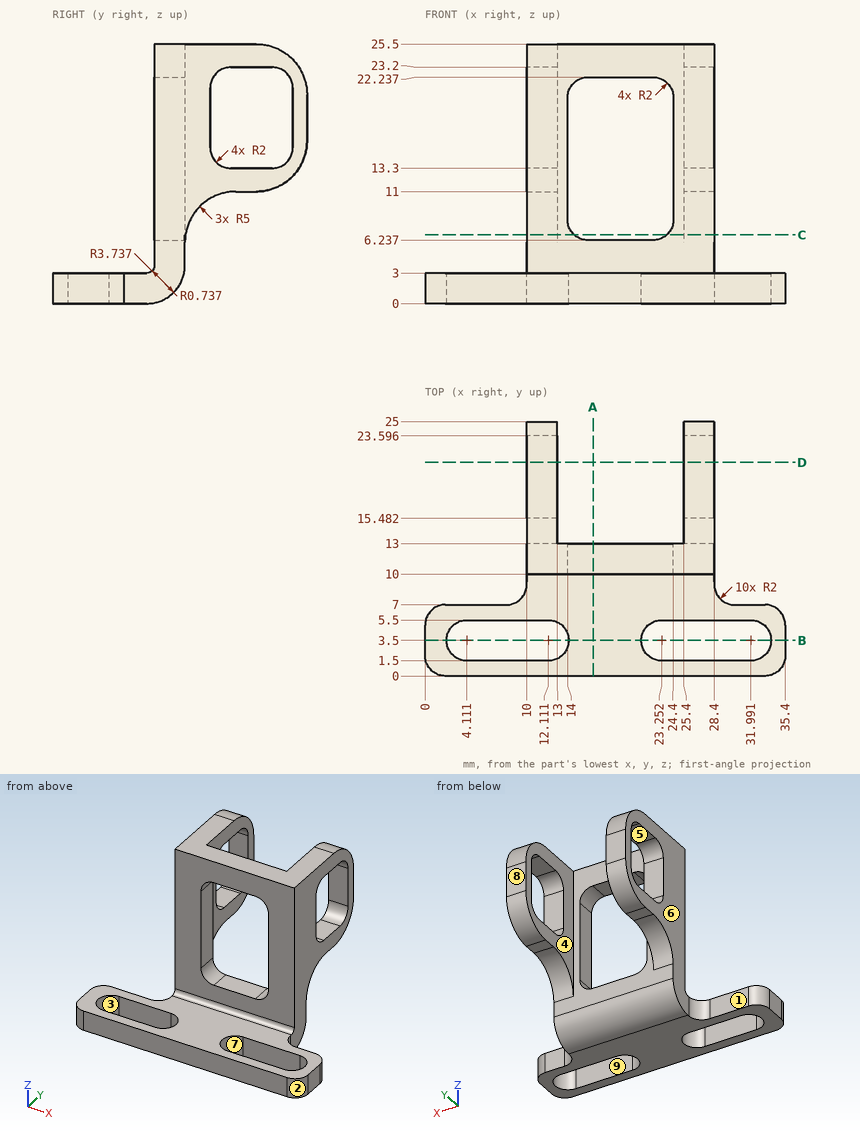
Input: dimensioned drawing with shaded views. Units: mm. Origin: part minimum x, y, z. A direction names the side the tool comes from. Round coordinates to 2 decimals unless told otherwise and drop trailing zeros. Order: outer loops, then holes, each group sorted by start corner. A loop starts at its lowest first (then second) coordinate and runs counter-clockwise, first axis right, second up.
1. Cut plane A-A, the plane x = 16.5. Output: boundary loops of the cut face in (y, z).
The answers:
outline: (0, 0) - (9.26, 0) arc R3.74 ccw to (13, 3.74) - (13, 6.24) - (10, 6.24) - (10, 3.74) arc R0.74 cw to (9.26, 3) - (0, 3) - close; (10, 22.24) - (13, 22.24) - (13, 25.5) - (10, 25.5) - close
2. Cut plane C-C, the plane z = 6.75. Output: boundary loops of the cut face in (x, y).
The answers:
outline: (10, 10) - (14.66, 10) - (14.66, 13) - (13, 13) - (13, 13.06) - (10, 13.06) - close; (23.74, 10) - (28.4, 10) - (28.4, 13.06) - (25.4, 13.06) - (25.4, 13) - (23.74, 13) - close
3. Cut plane D-D, the plane y = 21. Output: boundary loops of the cut face in (x, z), then the cut area to 3 significant figures.
The answers:
outline: (10, 11.1) - (13, 11.1) - (13, 13.3) - (10, 13.3) - close; (10, 23.2) - (13, 23.2) - (13, 25.4) - (10, 25.4) - close; (25.4, 11.1) - (28.4, 11.1) - (28.4, 13.3) - (25.4, 13.3) - close; (25.4, 23.2) - (28.4, 23.2) - (28.4, 25.4) - (25.4, 25.4) - close
area: 26.4 mm2
4. Mould query, pull axis X, two halves, no side actions, for the marked faces 6, 7, 8 and 9. Classes: released by +X, released by -X, zero draft, split by the parting line, or undercut.
The answers:
face 6: released by -X
face 7: undercut
face 8: zero draft
face 9: undercut
5. Set-up query: the marked faces 1, 2, 3, 4 and 5. Return all of +Z, -Z, +X, -X, +Y, -Y with unobstructed straight access to the full face (end or side cutting, diameter ignored); none if empty.
The answers:
face 1: +Z, -Z, -X, +Y
face 2: +Z, -Z, +X, -Y
face 3: +Z, -Z
face 4: +Z, -Z, +Y
face 5: +X, -X
6. Pin query (flat end, axial travel): P1, Ø3.5, axis at x = 5, z = 2, coming from the +Y side; P2, Ø5, axis at y = 11.5, z = 9, coming from the -X side; P3, Ø3.5, axis at y = 17, z = 15, coming from the +X side. Return the tip coordinate at first contact, or that it passes through.
The answers:
P1: stops at y = 7
P2: stops at x = 10
P3: stops at x = 28.4
7. Material intervals for line 1 (Y direction, x = 12, z = 19.25) (1 decimal); line 2 (X direction, y = 10.5, z = 16.5); line 3 (Z direction, x = 18.5, y = 8.5), sorted ascending.
The answers:
line 1: y = 10 to 15.5, 23.6 to 25
line 2: x = 10 to 14, 24.4 to 28.4
line 3: z = 0 to 3
8. Cut plane B-B, the plane y = 3.5. Output: boundary loops of the cut face in (x, z).
The answers:
outline: (0, 0) - (2.11, 0) - (2.11, 3) - (0, 3) - close; (14.11, 0) - (21.25, 0) - (21.25, 3) - (14.11, 3) - close; (33.99, 0) - (35.4, 0) - (35.4, 3) - (33.99, 3) - close
